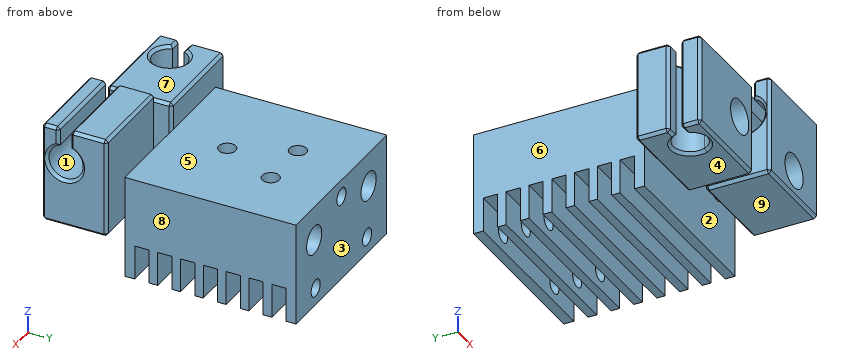
```python
from build123d import *

# Parameters (mm, degrees)
F0_W            = 30
F0_H            = 30
F11_DEPTH       = 18
F1_D            = 5
F1_DEPTH        = 20
F1_TIP          = 1.5021515476
F13_W           = 30
F13_H           = 2.5
F14_DEPTH       = 6
F15_D           = 3
F15_DEPTH       = 3
F15_TIP         = 0.9012909285
F16_D           = 3
F16_DEPTH       = 10
F16_TIP         = 0.9012909285
F3_R            = 1.475
F4_DEPTH        = 2.1
F18_W           = 17.5
F18_H           = 16
F17_W           = 16
F17_H           = 17.5
F19_DEPTH       = 11.4
F5_D            = 6
F5_DEPTH        = 5
F5_TIP          = 1.8025818571
F5_ON_F20_D     = 6
F5_ON_F20_DEPTH = 5
F5_ON_F20_TIP   = 1.8025818571
F8_DEPTH        = 16
F7_W            = 1.3441740274
F7_H            = 2
F22_DEPTH       = 16
F9_SIZE         = 0.49999


# Not quite as in the source:
# - a fillet or chamfer is up to 0.001 mm smaller than in the source, because OpenCascade refuses the exact size


with BuildPart() as f11:
    # F0 (on Top) → F11 (new body)
    with BuildSketch(Plane.XY):
        Rectangle(F0_W, F0_H)
    extrude(amount=F11_DEPTH)

    # F1
    with Locations(Plane(origin=(0, 15, 0), x_dir=(-1, 0, 0), z_dir=(0, 1, 0))):
        with Locations((-9, 12), (9, 12)):
            Hole(F1_D / 2, depth=F1_DEPTH)
            with Locations((0, 0, -(F1_DEPTH + F1_TIP / 2))):  # 118° drill point
                Cone(0, F1_D / 2, F1_TIP, mode=Mode.SUBTRACT)

    # F13 (on face) → F14 (cut)
    with BuildSketch(Plane(origin=(0, 0, 0), x_dir=(1, 0, 0), z_dir=(0, 0, -1))):
        with Locations((0, 12)):
            Rectangle(F13_W, F13_H)
        with Locations((0, 8)):
            Rectangle(F13_W, F13_H)
        with Locations((0, 4)):
            Rectangle(F13_W, F13_H)
        Rectangle(F13_W, F13_H)
        with Locations((0, -4)):
            Rectangle(F13_W, F13_H)
        with Locations((0, -8)):
            Rectangle(F13_W, F13_H)
        with Locations((0, -12)):
            Rectangle(F13_W, F13_H)
    extrude(amount=-F14_DEPTH, mode=Mode.SUBTRACT)

    # F15
    with Locations(Plane.XY.offset(18)):
        with Locations((4.5, 5), (-4.5, 5), (0, -5)):
            Hole(F15_D / 2, depth=F15_DEPTH)
            with Locations((0, 0, -(F15_DEPTH + F15_TIP / 2))):  # 118° drill point
                Cone(0, F15_D / 2, F15_TIP, mode=Mode.SUBTRACT)

    # F16
    with Locations(Plane(origin=(0, 15, 0), x_dir=(-1, 0, 0), z_dir=(0, 1, 0))):
        with Locations((8.5, 3), (-8.5, 3), (0, 15)):
            Hole(F16_D / 2, depth=F16_DEPTH)
            with Locations((0, 0, -(F16_DEPTH + F16_TIP / 2))):  # 118° drill point
                Cone(0, F16_D / 2, F16_TIP, mode=Mode.SUBTRACT)

    # F3 (on face) → F4 (join)
    with BuildSketch(Plane.XZ.offset(15)):
        with Locations((-9, 12)):
            Circle(F3_R)
        with Locations((9, 12)):
            Circle(F3_R)
    extrude(amount=F4_DEPTH)

    # F18 (on face) + F17 (on face) → F19 (join)
    with BuildSketch(Plane.XZ.offset(17.1)):
        with Locations((-13.25, 12)):
            Rectangle(F18_W, F18_H)
    with BuildSketch(Plane.XZ.offset(17.1)):
        with Locations((9, 16.25)):
            Rectangle(F17_W, F17_H)
    extrude(amount=F19_DEPTH)

    # F5
    with Locations(Plane.XZ.offset(28.5)):
        with Locations((-9, 12)):
            Hole(F5_D / 2, depth=F5_DEPTH)
            with Locations((0, 0, -(F5_DEPTH + F5_TIP / 2))):  # 118° drill point
                Cone(0, F5_D / 2, F5_TIP, mode=Mode.SUBTRACT)

    # F5 on F20
    with Locations(Plane.XZ.offset(28.5)):
        with Locations((9, 12)):
            Hole(F5_ON_F20_D / 2, depth=F5_ON_F20_DEPTH)
            with Locations((0, 0, -(F5_ON_F20_DEPTH + F5_ON_F20_TIP / 2))):  # 118° drill point
                Cone(0, F5_ON_F20_D / 2, F5_ON_F20_TIP, mode=Mode.SUBTRACT)

    # F6 (on face) → F8 (cut, through all)
    with BuildSketch(Plane.YZ.offset(17)):
        with BuildLine():
            Line((-25.5, 25), (-25.5, 21.7284271247))
            ThreePointArc((-25.5, 21.7284271247), (-24.5, 15.9), (-23.5, 21.7284271247))
            Line((-23.5, 21.7284271247), (-23.5, 25))
            Line((-23.5, 25), (-25.5, 25))
        make_face()
    extrude(amount=-F8_DEPTH, mode=Mode.SUBTRACT)

    # F7 (on face) → F22 (cut, through all)
    with BuildSketch(Plane.XY.offset(20)):
        with BuildLine():
            Line((-22, -24.9799899757), (-19.6726011522, -24.9799899757))
            ThreePointArc((-19.6726011522, -24.9799899757), (-16.8441740274, -26.9799899757), (-14.0157469027, -24.9799899757))
            ThreePointArc((-14.0157469027, -24.9799899757), (-15.8441740274, -21.1515628509), (-19.6726011522, -22.9799899757))
            Line((-19.6726011522, -22.9799899757), (-22, -22.9799899757))
            Line((-22, -22.9799899757), (-22, -24.9799899757))
        make_face()
        with Locations((-22.6720870137, -23.9799899757)):
            Rectangle(F7_W, F7_H)
    extrude(amount=-F22_DEPTH, mode=Mode.SUBTRACT)

    # F9 (size 0.5 in the source; OpenCascade refuses exactly that, so slightly less here)
    f9_edges = [f11.edges().sort_by_distance(p)[0] for p in [
        (17, -17.1, 16.25),
        (17, -20.3, 25),
        (17, -23.5, 23.364214),
        (17, -24.5, 15.9),
        (17, -25.5, 23.364214),
        (17, -27, 25),
        (17, -28.5, 16.25),
        (17, -22.8, 7.5),
        (1, -22.8, 7.5),
        (9, -17.1, 7.5),
        (9, -28.5, 7.5),
        (-13.25, -17.1, 4),
        (-4.5, -22.8, 4),
        (-13.25, -28.5, 4),
        (-22, -26.739995, 4),
        (-20.836301, -24.97999, 4),
        (-13.844174, -23.97999, 4),
        (-20.836301, -22.97999, 4),
        (-22, -20.039995, 4),
        (-4.5, -22.8, 20),
        (-4.5, -17.1, 12),
        (-4.5, -28.5, 12),
        (9, -17.1, 25),
        (1, -20.3, 25),
        (9, -23.5, 25),
        (9, -25.5, 25),
        (1, -27, 25),
        (9, -28.5, 25),
        (-13.25, -17.1, 20),
        (-22, -20.039995, 20),
        (-20.836301, -22.97999, 20),
        (-13.844174, -23.97999, 20),
        (-20.836301, -24.97999, 20),
        (-22, -26.739995, 20),
        (-13.25, -28.5, 20),
        (-22, -17.1, 12),
        (-22, -22.97999, 12),
        (1, -17.1, 16.25),
        (1, -28.5, 16.25),
        (1, -25.5, 23.364214),
        (1, -24.5, 15.9),
        (1, -23.5, 23.364214),
        (-22, -24.97999, 12),
        (-22, -28.5, 12),
    ]]
    chamfer(f9_edges, length=F9_SIZE)


solid = f11.part
```
Build history of the part. All positions in model axes, mm. Face numbers are marked on the shaded views. A direction names the side the tool comes from. Round coordinates to 2 decimals unless told otherwise and drop trailing zeros. Loops run counter-clockwise (first coordinate to the right, second up) from the corner with the lowest first, then second, coordinate; pieces in that order, holes last.
Item 1: Two-plate mould, pull along Y, no slides. Class the marked faces 1, 2, 3 and 4: released by +Y, released by -Y, zero draft, split by the parting line, or undercut.
Item 2: Drill centre lines: line 1 along X through (y, z) = (5, 16.8); line 2 along X through (y, z) = (11.25, 12); line 3 along Z through (x, y) = (-9, -25.45). Where is each one in solid material? Low to high.
Item 3: Saw through at B-B (y = 0). List the corners of the cut face in (x, z), then the cut area to 3 significant figures.
Item 4: Saw through at C-C (y = 7.5). List the corners of the cut face in (x, z).
Item 5: Saw through at A-A (z = 18.9). State how many separate pieces and enclosed holes the cut face has, then the cut area to 3 significant figures.
Item 6: Which spindle directions (+Z, -Z, +X, -X, +Y, -Y) get a long thin tool onto all of the face, cutting with end or side? Do the marked faces 5, 6, 7, 8 and 9. Say none if no direction does.
Item 7: Pin check, flat tips, straight feed: P1, Ø1, axis at y = 3, z = 12.5, coming from the -X side; P2, Ø1.8, axis at x = -1, z = 4, coming from the -Y side; P3, Ø10, axis at x = 12.5, y = 5, coming from the +Z side. Stop position of each tip, or through.
Worked answers:
1. face 1: undercut
1. face 2: undercut
1. face 3: released by +Y
1. face 4: zero draft
2. line 1: x = -15 to -6, -3 to 3, 6 to 15
2. line 2: x = -15 to -11.5, -6.5 to 6.5, 11.5 to 15
2. line 3: z = 4 to 9, 15 to 20
3. outline: (-15, 6) - (15, 6) - (15, 18) - (-15, 18) - close; hole circle Ø5 at (-9, 12); hole circle Ø5 at (9, 12)
3. area: 321 mm2
4. outline: (-15, 6) - (15, 6) - (15, 18) - (-15, 18) - close; hole circle Ø5 at (-9, 12); hole circle Ø3 at (0, 15); hole circle Ø5 at (9, 12)
5. separate pieces: 3
5. enclosed holes: 0
5. area: 251 mm2
6. face 5: +Z, +X, -X, +Y
6. face 6: +Z, -Z, -X, +Y
6. face 7: +Z, -X, +Y, -Y
6. face 8: +Z, -Z, +X, +Y
6. face 9: -Z, +X, -Y
7. P1: stops at x = -15
7. P2: stops at y = -15
7. P3: stops at z = 18
